Autodesk Inventor part; units mm, degrees
ref_plane "YZ Plane" through (0, 0, 0) normal (1, 0, 0) x (0, 1, 0)
ref_plane "XZ Plane" through (0, 0, 0) normal (0, 1, 0) x (-1, 0, 0)
ref_plane "XY Plane" through (0, 0, 0) normal (0, 0, 1) x (1, 0, 0)
sketch "Sketch1" plane through (0, 0, 0) normal (0, 1, 0) x (-1, 0, 0)
  line L0 (-76.2, 50.8) -> (76.2, 50.8)
  line L1 (76.2, 50.8) -> (76.2, -50.8)
  line L2 (76.2, -50.8) -> (-76.2, -50.8)
  line L3 (-76.2, -50.8) -> (-76.2, 50.8)
  line L4 (-76.2, 50.8) -> (76.2, -50.8) construction
  line L5 (76.2, 50.8) -> (-76.2, -50.8) construction
  point P0 (0, 0)
  dimension "d0" = 152.4
  dimension "d1" = 101.6
extrude "Extrusion1" add sketch "Sketch1" along normal blind 2.032
sketch "Sketch2" plane through (0, 2.032, 0) normal (0, 1, 0) x (1, 0, 0)
  line L0 (-76.2, -50.8) -> (76.2, -50.8)
  line L1 (76.2, -50.8) -> (76.2, 50.8)
  line L2 (-76.2, -50.8) -> (76.2, -50.8)
  line L3 (76.2, -50.8) -> (76.2, 50.8)
  line L4 (76.2, 50.8) -> (-76.2, 50.8)
  line L5 (-76.2, 50.8) -> (-76.2, -50.8)
  line L6 (75.184, -49.784) -> (-75.184, -49.784)
  line L7 (-75.184, -49.784) -> (-75.184, 49.784)
  line L8 (-75.184, 49.784) -> (75.184, 49.784)
  line L9 (75.184, 49.784) -> (75.184, -49.784)
  line L10 (75.184, -49.784) -> (-75.184, 49.784) construction
  line L11 (-75.184, -49.784) -> (75.184, 49.784) construction
  point P0 (0, 0)
  dimension "d4" = 150.368
  dimension "d5" = 99.568
extrude "Extrusion2" add sketch "Sketch2" along normal blind 76.2
sketch "Sketch3" plane through (0, 2.032, 0) normal (0, 1, 0) x (1, 0, 0)
  circle A0 centre (0, -25.4) radius 2.0828
  circle A1 centre (0, 25.4) radius 2.0828
  point P0 (0, 0)
  dimension "d10" = 4.1656
  dimension "d11" = 4.1656
extrude "Extrusion3" cut sketch "Sketch3" against normal through all
properties part number "546-1444-8-6x4-Enclosure"
Design review of the part built by this model. Coordinates are the model's own, in mm. A direction names the side the tool comes from. Round coordinates to 2 decimals unless told otherwise and drop trailing zeros. Write each loop counter-clockwise with the first axis right and the second up, starting at its lowest first coordinate (ties: lowest second). Pieces come first, ordered by that corner, then holes. Notation, with made-up numbers: (-21.75, 62) -> (26.25, 62) arc R19 cw to (26.25, 73) -> close; hole circle Ø7 at (50.5, 49). An arc over 180 degrees is marked (long way). One line per item, written item: value. Start each with the question number.
Q1. Add section A-A (x = 0). Give the boundary of the cut face in (y, z).
Q2. The part is to be moulded in two halves that separate along Y. For faces 1 (the face through (1, 2.032, 1)), 2 (the face through (-1, 39, -50.8)), 3 (the face through (1, 0, 1)), say which applies: pulls with the +Y half, pulls with the -Y half, needs draft (parallel to the pull), parting line crosses it, or undercut.
Q3. Add section D-D (z = -4). Give the boundary of the cut face in (x, y), then the cut area to 3 significant figures.
Q4. Add section B-B (z = -25.4). Give the boundary of the cut face in (x, y), then the cut area to 3 significant figures.
Q5. Insertion check: P1, Ø5, axis at x = 0, z = -25.4, coming from the +Y side. The pin has a flat end and moves straight along its axis. Give the tip position at first contact, or say it passes through.
Q6. Add section C-C (y = 14). Give the boundary of the cut face in (x, z), then the cut area to 3 significant figures.
Q7. To check wall thickness, follow probe 1 along Z at (x, y) = (0, 1); probe 2 along Z at (x, y) = (0, 6.5); probe 3 along X at (y, z) = (1, -25). State the ranges of each line that lie inside material, in increasing order.
Q8. Tool access review of faces 4 (the face through (-76.2, 39, 1)), 5 (the face through (75.184, 40, -1)): name each direction out of +Z, -Z, +X, -X, +Y, -Y from which nothing blocks a thin tool from reaching the whole face with its end or side.
Response:
1. outline: (0, -50.8) -> (78.23, -50.8) -> (78.23, -49.78) -> (2.03, -49.78) -> (2.03, -27.48) -> (0, -27.48) -> close; (0, -23.32) -> (2.03, -23.32) -> (2.03, 23.32) -> (0, 23.32) -> close; (0, 27.48) -> (2.03, 27.48) -> (2.03, 49.78) -> (78.23, 49.78) -> (78.23, 50.8) -> (0, 50.8) -> close
2. face 1: pulls with the +Y half
2. face 2: needs draft
2. face 3: pulls with the -Y half
3. outline: (-76.2, 0) -> (76.2, 0) -> (76.2, 78.23) -> (75.18, 78.23) -> (75.18, 2.03) -> (-75.18, 2.03) -> (-75.18, 78.23) -> (-76.2, 78.23) -> close
3. area: 465 mm^2
4. outline: (-76.2, 0) -> (-2.08, 0) -> (-2.08, 2.03) -> (-75.18, 2.03) -> (-75.18, 78.23) -> (-76.2, 78.23) -> close; (2.08, 0) -> (76.2, 0) -> (76.2, 78.23) -> (75.18, 78.23) -> (75.18, 2.03) -> (2.08, 2.03) -> close
4. area: 456 mm^2
5. P1: stops at y = 2.03
6. outline: (-76.2, -50.8) -> (76.2, -50.8) -> (76.2, 50.8) -> (-76.2, 50.8) -> close; hole (-75.18, -49.78) -> (75.18, -49.78) -> (75.18, 49.78) -> (-75.18, 49.78) -> close
6. area: 512 mm^2
7. probe 1: z = -50.8 to -27.48, -23.32 to 23.32, 27.48 to 50.8
7. probe 2: z = -50.8 to -49.78, 49.78 to 50.8
7. probe 3: x = -76.2 to -2.04, 2.04 to 76.2
8. face 4: +Z, -Z, -X, +Y, -Y
8. face 5: +Y
